Check sheet for the drawn part. Datum: minimum x, y, z corner. Units: mm. Round coordinates to 2 decimals unless told otherwise and drop trailing zeros. Write each loop counter-clockwise with the first axis right and the second up, starting at its lowest first coordinate (ties: lowest second). Pieces come first, ordered by that corner, then holes.
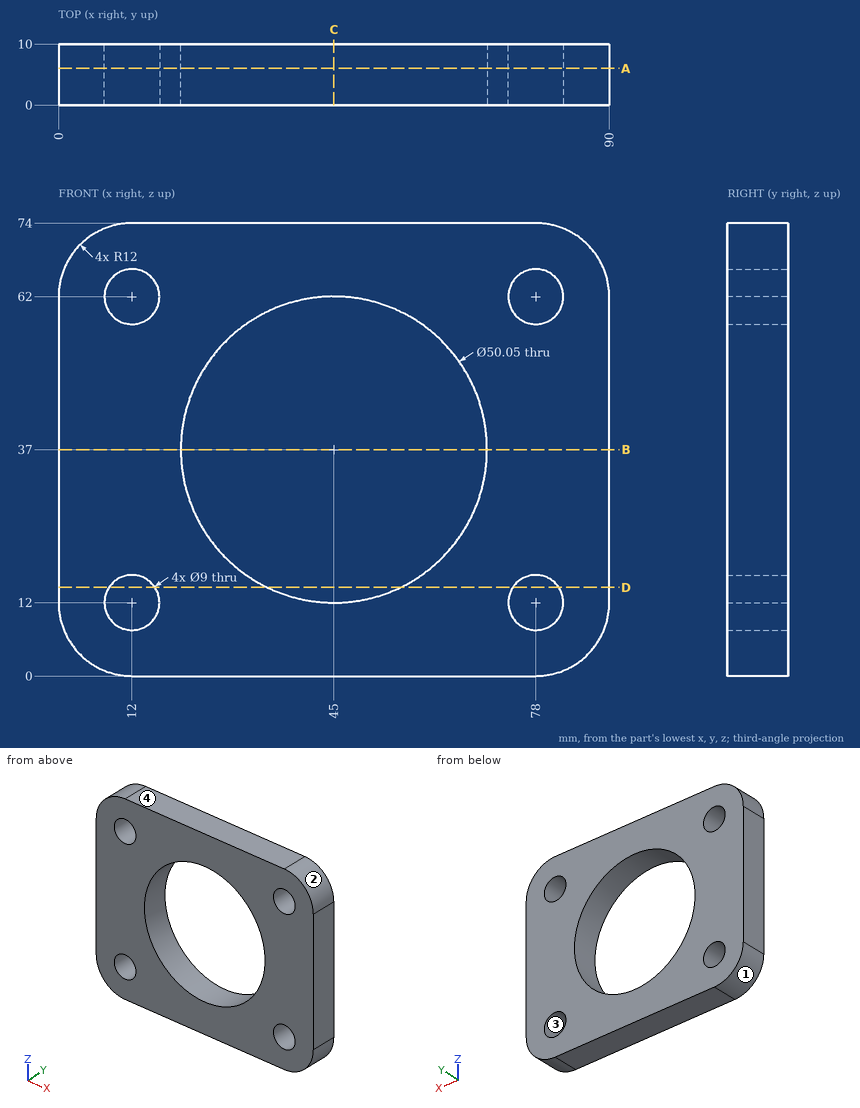
Q1. Sectioned sample at D-D (z = 14.5). Enter the section's corners in (x, y), plus the area to 3 significant figures.
Recorded:
outline: (0, 0) - (8.26, 0) - (8.26, 10) - (0, 10) - close; (15.74, 0) - (34.05, 0) - (34.05, 10) - (15.74, 10) - close; (55.95, 0) - (74.26, 0) - (74.26, 10) - (55.95, 10) - close; (81.74, 0) - (90, 0) - (90, 10) - (81.74, 10) - close
area: 531 mm2
Q2. Sectioned sample at A-A (y = 6). Enter the section's corners in (x, z) (3 decimals).
Recorded:
outline: (0, 12) arc R12 ccw to (12, 0) - (78, 0) arc R12 ccw to (90, 12) - (90, 62) arc R12 ccw to (78, 74) - (12, 74) arc R12 ccw to (0, 62) - close; hole circle Ø9 at (12, 12); hole circle Ø9 at (12, 62); hole circle Ø50.05 at (45, 37); hole circle Ø9 at (78, 12); hole circle Ø9 at (78, 62)
Q3. Material ranges on line 1 along Z through (x, y) = (78, 5.75); line 2 along X through (y, z) = (4.5, 37.5); line 3 along Z through (x, y) = (63.5, 3), recorded low to high.
Recorded:
line 1: z = 0 to 7.5, 16.5 to 57.5, 66.5 to 74
line 2: x = 0 to 19.98, 70.02 to 90
line 3: z = 0 to 20.15, 53.85 to 74
Q4. Sectioned sample at B-B (z = 37). Enter the section's corners in (x, y) (3 decimals).
Recorded:
outline: (0, 0) - (19.975, 0) - (19.975, 10) - (0, 10) - close; (70.025, 0) - (90, 0) - (90, 10) - (70.025, 10) - close
Q5. Depth check by flat-ended pin: P1, Ø7, axis at x = 78, z = 12, coming from the +Y side; P2, Ø4, axis at y = 3, z = 7.5, coming from the -X side. Enter the tip coordinate at first touch or a pass-through.
Recorded:
P1: passes through
P2: stops at x = 0.26
Q6. Sectioned sample at C-C (x = 45). Enter the section's corners in (y, z) (3 decimals).
Recorded:
outline: (0, 0) - (10, 0) - (10, 11.975) - (0, 11.975) - close; (0, 62.025) - (10, 62.025) - (10, 74) - (0, 74) - close
Q7. Release check for a two-part mould opening along X. For the marked faces 1, 2, 3 and 4 record: released by +X, released by -X, zero draft, split by the parting line, or undercut.
Recorded:
face 1: released by -X
face 2: released by +X
face 3: undercut
face 4: zero draft
